Verification items for the finished model (mm, model axes). Face numbers are marked on the shaded views. A direction names the side the tool comes from. Give positions to 0.01 mm unless a question says otherwise; leave off trailing zeros. Order: outer loops, then holes, each group sorted by start corner. A loop starts at its lowest first (then second) coordinate and runs counter-clockwise, first axis right, second up. Notation, with made-up numbers: (-11, 88.5) -> (5, 88.5) arc R31 cw to (5, 112.5) -> close; hole circle Ø11 at (84.5, 24). An arc over 180 degrees is marked (long way). Return JSON: item names as keys, results as strings. Group by question number.
(1) Tool access check on the marked faces 1 and 2. Record the directions out of +Z, -Z, +X, -X, +Y, -Y that give a thin tool (end or side, any length) a straight path to the whole face; none if there is none.
(2) Cross-section at A-A on x = 9.5. Enter the section's corners in (y, z).
(3) Depth check by flat-ended pin: pin 1 Ø8 at (x, z) = (18.5, 5) entering from +Y; pin 2 Ø4 at (x, z) = (31, -2) entering from +Y; pin 3 Ø1.5 at (x, z) = (7, 6.5) entering from +Y. Enter the tip coordinate at first touch or a pass-through.
(4) Thickness scan on line 1 along X through (y, z) = (-4.25, -5.75); line 2 along Y through (x, z) = (6.5, -4.5); line 3 along Z through (x, y) = (29.5, 3.25). Record the ranges inside material, lowest first.
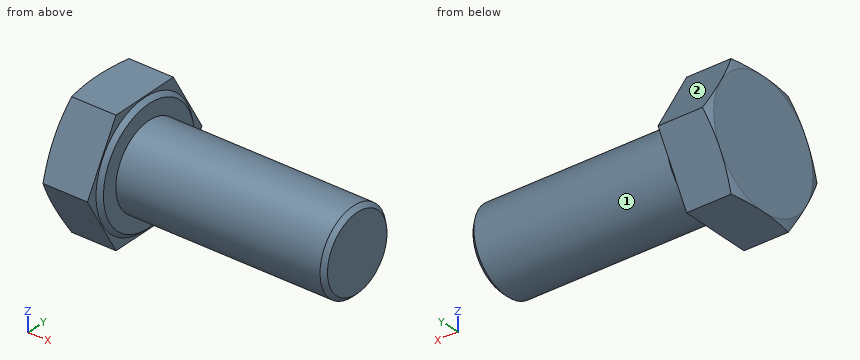
from build123d import *

# Parameters (mm, degrees)
BASEHEAD_DEPTH = 7.5
SKETCH5_R      = 6
BASEBODY_DEPTH = 30
CHAMFER1_SIZE  = 0.6


with BuildPart() as part:
    # Sketch2 → BaseHead (new body)
    with BuildSketch(Plane(origin=(0, 0, 0), x_dir=(0, 0, -1), z_dir=(1, 0, 0))):
        Polygon((0, -10.392304845), (9, -5.196152423), (9, 5.196152423), (0, 10.392304845), (-9, 5.196152423), (-9, -5.196152423), align=None)
    extrude(amount=BASEHEAD_DEPTH)

    # Sketch3 → BearingFace (revolve, cut)
    with BuildSketch(Plane.XY, mode=Mode.PRIVATE) as bearingface_sk:
        Polygon((7.5, 10.392304845), (7.5, 8.235), (6.9, 8.835), (6.9, 10.392304845), align=None)
    revolve(bearingface_sk.sketch.rotate(Axis((-0.957090588, 0, 0), (1, 0, 0)), 90), axis=Axis((-0.957090588, 0, 0), (1, 0, 0)), mode=Mode.SUBTRACT)

    # Sketch4 → HeadChamfer (revolve, cut)
    with BuildSketch(Plane.XY):
        Polygon((0, 10.392304845), (0.506757521, 10.392304845), (0, 9), align=None)
    revolve(axis=Axis((-0.493528746, 0, 0), (1, 0, 0)), mode=Mode.SUBTRACT)

    # Sketch5 → BaseBody (add)
    with BuildSketch(Plane(origin=(7.5, 0, 0), x_dir=(0, 0, -1), z_dir=(1, 0, 0))):
        Circle(SKETCH5_R)
    extrude(amount=BASEBODY_DEPTH)

    # Chamfer1
    chamfer1_edges = [part.edges().sort_by_distance(p)[0] for p in [
        (37.5, 0, 6),
    ]]
    chamfer(chamfer1_edges, length=CHAMFER1_SIZE)


solid = part.part
Verdict:
{
 "1": {"face 1": "+X", "face 2": "+Z, +X, -X, +Y"},
 "2": {"outline": "circle Ø12 at (0, 0)"},
 "3": {"pin 1": "y = 5.92", "pin 2": "y = 6", "pin 3": "y = 7.07"},
 "4": {"line 1": "0 to 7.5", "line 2": "-7.79 to 7.79", "line 3": "-5.04 to 5.04"}
}
